```python
from build123d import *

# Parameters (mm, degrees)
BASE_FLANGE1_DEPTH           = 3
EDGE_FLANGE1_STRIP_W         = 13.4732
EDGE_FLANGE1_STRIP_H         = 3
EDGE_FLANGE1_STRIP_CUT_DEPTH = 56
EDGE_FLANGE1_DEPTH           = 56
EDGE_FLANGE1_FLAT_DEPTH      = 3
SKETCH5_R                    = 2.25
CUT_EXTRUDE1_DEPTH           = 3
CHAMFER1_SIZE                = 2


# Sheet-metal steps are written as plain solids
with BuildPart() as part:
    # Sketch1 → Base-Flange1 (new body)
    with BuildSketch(Plane(origin=(0, 0, 0), x_dir=(1, 0, 0), z_dir=(0, 1, 0))):
        with BuildLine():
            Line((-18.5, 28), (15.5, 28))
            ThreePointArc((15.5, 28), (17.621320344, 27.121320344), (18.5, 25))
            Line((18.5, 25), (18.5, -25))
            ThreePointArc((18.5, -25), (17.621320344, -27.121320344), (15.5, -28))
            Line((15.5, -28), (-18.5, -28))
            Line((-18.5, -28), (-18.5, 28))
        make_face()
        with BuildLine():
            Line((-7.5, -15.25), (12.5, -15.25))
            ThreePointArc((12.5, -15.25), (15.25, -18), (12.5, -20.75))
            Line((12.5, -20.75), (-7.5, -20.75))
            ThreePointArc((-7.5, -20.75), (-10.25, -18), (-7.5, -15.25))
        make_face(mode=Mode.SUBTRACT)
        with BuildLine():
            Line((-7.5, 15.25), (12.5, 15.25))
            ThreePointArc((12.5, 15.25), (15.25, 18), (12.5, 20.75))
            Line((12.5, 20.75), (-7.5, 20.75))
            ThreePointArc((-7.5, 20.75), (-10.25, 18), (-7.5, 15.25))
        make_face(mode=Mode.SUBTRACT)
    extrude(amount=-BASE_FLANGE1_DEPTH)

    # Edge-Flange1 strip (across the edge) → Edge-Flange1 strip cut (cut)
    with BuildSketch(Plane(origin=(-18.5, 0, -28), x_dir=(1, 0, 0), z_dir=(0, 0, 1))):
        with Locations((-3, -1.5)):
            Rectangle(EDGE_FLANGE1_STRIP_W, EDGE_FLANGE1_STRIP_H)
    extrude(amount=EDGE_FLANGE1_STRIP_CUT_DEPTH, mode=Mode.SUBTRACT)

    # Edge-Flange1 bend section (across the edge) → Edge-Flange1 (add)
    with BuildSketch(Plane(origin=(-18.5, 0, -28), x_dir=(1, 0, 0), z_dir=(0, 0, 1))):
        with BuildLine():
            Line((0, 0.7366), (3, 0.7366))
            ThreePointArc((3, 0.7366), (3.215745145, 0.215745145), (3.7366, 0))
            Line((3.7366, 0), (3.7366, -3))
            ThreePointArc((3.7366, -3), (1.094424801, -1.905575199), (0, 0.7366))
        make_face()
    extrude(amount=EDGE_FLANGE1_DEPTH)

    # Edge-Flange1 profile (on flange) → Edge-Flange1 flat (add)
    with BuildSketch(Plane(origin=(-18.5, 0, 0), x_dir=(0, 0, -1), z_dir=(1, 0, 0))):
        with BuildLine():
            Line((-28, 0.7366), (28, 0.7366))
            Line((28, 0.7366), (28, 44))
            ThreePointArc((28, 44), (27.121320344, 46.121320344), (25, 47))
            Line((25, 47), (-25, 47))
            ThreePointArc((-25, 47), (-27.121320344, 46.121320344), (-28, 44))
            Line((-28, 44), (-28, 0.7366))
        make_face()
    extrude(amount=EDGE_FLANGE1_FLAT_DEPTH)

    # Sketch5 → Cut-Extrude1 (cut)
    with BuildSketch(Plane.ZY.offset(18.5)):
        with BuildLine():
            Line((9, 37), (-9, 37))
            ThreePointArc((-9, 37), (-11.565163819, 36.665398832), (-13.958666275, 35.683986917))
            Line((-13.958666275, 35.683986917), (-15.155612761, 37.120322699))
            ThreePointArc((-15.155612761, 37.120322699), (-16.195875666, 37.723371228), (-17.379716482, 37.512811591))
            ThreePointArc((-17.379716482, 37.512811591), (-17.498601644, 37.426573777), (-17.620322699, 37.344387239))
            ThreePointArc((-17.620322699, 37.344387239), (-18.242813111, 36.158437556), (-17.844387239, 34.879677301))
            Line((-17.844387239, 34.879677301), (-16.647440754, 33.443341518))
            ThreePointArc((-16.647440754, 33.443341518), (-19, 27), (-16.647440754, 20.556658482))
            Line((-16.647440754, 20.556658482), (-17.844387239, 19.120322699))
            ThreePointArc((-17.844387239, 19.120322699), (-18.242813111, 17.841562444), (-17.620322699, 16.655612761))
            ThreePointArc((-17.620322699, 16.655612761), (-17.498601644, 16.573426223), (-17.379716482, 16.487188409))
            ThreePointArc((-17.379716482, 16.487188409), (-16.195875666, 16.276628772), (-15.155612761, 16.879677301))
            Line((-15.155612761, 16.879677301), (-13.958666275, 18.316013083))
            ThreePointArc((-13.958666275, 18.316013083), (-11.565163819, 17.334601168), (-9, 17))
            Line((-9, 17), (9, 17))
            ThreePointArc((9, 17), (11.565163819, 17.334601168), (13.958666275, 18.316013083))
            Line((13.958666275, 18.316013083), (15.155612761, 16.879677301))
            ThreePointArc((15.155612761, 16.879677301), (16.195875666, 16.276628772), (17.379716482, 16.487188409))
            ThreePointArc((17.379716482, 16.487188409), (17.498601644, 16.573426223), (17.620322699, 16.655612761))
            ThreePointArc((17.620322699, 16.655612761), (18.242813111, 17.841562444), (17.844387239, 19.120322699))
            Line((17.844387239, 19.120322699), (16.647440754, 20.556658482))
            ThreePointArc((16.647440754, 20.556658482), (19, 27), (16.647440754, 33.443341518))
            Line((16.647440754, 33.443341518), (17.844387239, 34.879677301))
            ThreePointArc((17.844387239, 34.879677301), (18.242813111, 36.158437556), (17.620322699, 37.344387239))
            ThreePointArc((17.620322699, 37.344387239), (17.498601644, 37.426573777), (17.379716482, 37.512811591))
            ThreePointArc((17.379716482, 37.512811591), (16.195875666, 37.723371228), (15.155612761, 37.120322699))
            Line((15.155612761, 37.120322699), (13.958666275, 35.683986917))
            ThreePointArc((13.958666275, 35.683986917), (11.565163819, 36.665398832), (9, 37))
        make_face()
        with Locations(Location((20, 41, 0), (0, 0, 270))):
            Circle(SKETCH5_R)
        with Locations(Location((-20, 41, 0), (0, 0, 270))):
            Circle(SKETCH5_R)
        with Locations(Location((-20, 13, 0), (0, 0, 270))):
            Circle(SKETCH5_R)
        with Locations(Location((20, 13, 0), (0, 0, 270))):
            Circle(SKETCH5_R)
    extrude(amount=-CUT_EXTRUDE1_DEPTH, mode=Mode.SUBTRACT)

    # Chamfer1
    chamfer1_edges = [part.edges().sort_by_distance(p)[0] for p in [
        (-18.5, 15.25, -20),
        (-18.5, 15.25, 20),
        (-18.5, 43.25, 20),
        (-18.5, 43.25, -20),
    ]]
    chamfer(chamfer1_edges, length=CHAMFER1_SIZE)


solid = part.part
```
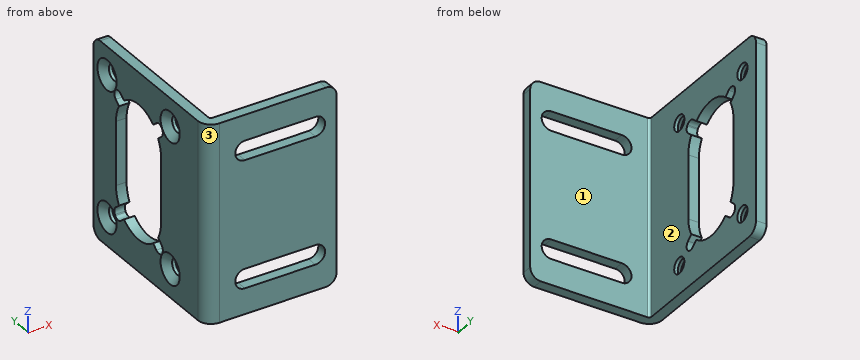
Design review of the part built by this model. Coordinates are the model's own, in mm. Face numbers are marked on the shaded views. Coordinates: 2 decimals unless noted, no trailing zeros. Loops run counter-clockwise (first coordinate to the right, second up) from the corner with the lowest first, then second, coordinate; pieces in that order, holes last.
Q1. For pin 1 (0.9 mm diameter, centred on x = -16.5, z = 4.5, fed in from -Y); pin 2 (5 mm diameter, centred on y = 41, z = 20, fed in from -X); pin 3 (3.5 mm diameter, centred on y = 41, z = -20, fed in from -X); pin 4 (1 mm diameter, centred on y = 2.5, z = -9, fed in from +X), all flat-tipped, find the tip position at first contact; note any pin that passes through.
Reported:
pin 1: stops at y = -2.77
pin 2: stops at x = -16.75
pin 3: passes through
pin 4: stops at x = -15.5
Q2. We need section A-A on z = -4.5. State the section outline as (x, y) points, and give its area (3 significant figures).
Reported:
outline: (-18.5, 0.74) arc R3.74 ccw to (-14.76, -3) - (18.5, -3) - (18.5, 0) - (-14.76, 0) arc R0.74 cw to (-15.5, 0.74) - (-15.5, 17) - (-18.5, 17) - close; (-18.5, 37) - (-15.5, 37) - (-15.5, 47) - (-18.5, 47) - close
area: 189 mm2
Q3. We need section B-B on x = 3.5. State the section outline as (y, z) points.
Reported:
outline: (-3, -28) - (0, -28) - (0, -20.75) - (-3, -20.75) - close; (-3, -15.25) - (0, -15.25) - (0, 15.25) - (-3, 15.25) - close; (-3, 20.75) - (0, 20.75) - (0, 28) - (-3, 28) - close
Q4. We need section C-C on y = 13. State the section outline as (x, z) points.
Reported:
outline: (-18.5, -28) - (-15.5, -28) - (-15.5, -22.25) - (-16.5, -22.25) - (-18.5, -24.25) - close; (-18.5, -15.75) - (-16.5, -17.75) - (-15.5, -17.75) - (-15.5, 17.75) - (-16.5, 17.75) - (-18.5, 15.75) - close; (-18.5, 24.25) - (-16.5, 22.25) - (-15.5, 22.25) - (-15.5, 28) - (-18.5, 28) - close
Q5. We need section D-D on y = 21.5. State the section outline as (x, z) points, and give its area (3 significant figures).
Reported:
outline: (-18.5, -28) - (-15.5, -28) - (-15.5, -17.35) - (-18.5, -17.35) - close; (-18.5, 17.35) - (-15.5, 17.35) - (-15.5, 28) - (-18.5, 28) - close
area: 63.9 mm2
Q6. To check wall thickness, follow line 1 (Z direction, x = -17, y = 12); line 2 (X direction, y = 32, z = 19); line 3 (Y direction, x = 6.5, z = 1). State the ranges of each line that lie inside material, in increasing order.
Reported:
line 1: z = -28 to -22.56, -17.44 to 17.44, 22.56 to 28
line 2: x = -18.5 to -15.5
line 3: y = -3 to 0
Q7. The part is to be moulded in two halves that separate along X. For the marked faces 1, 2 and 3, say which applies: +X half, -X half, draft (parallel to the pull), parting line (faces both ways), or undercut.
Reported:
face 1: draft
face 2: +X half
face 3: -X half
